For this review, take the finished solid that the model builds, in its own axes (mm). A direction names the side the tool comes from. Round coordinates to 2 decimals unless told otherwise and drop trailing zeros. Loops run counter-clockwise (first coordinate to the right, second up) from the corner with the lowest first, then second, coordinate; pieces in that order, holes last. Notation, with made-up numbers: M 19.5,-21.5 L 62.5,-21.5 A28 cw 62.5,10.5 Z; hole C 23.25,68 d10. An arc over 180 degrees is marked long. Write item = value, one per line. Start each with the question number.
```python
from build123d import *

# Parameters (mm, degrees)
SKETCH1_W               = 119
SKETCH1_H               = 50
BOSS_EXTRUDE1_DEPTH     = 95
SKETCH2_W               = 115
SKETCH2_H               = 46
CUT_EXTRUDE1_DEPTH      = 92
SKETCH3_W               = 50
SKETCH3_H               = 29
CUT_EXTRUDE2_DEPTH      = 10
SKETCH4_R               = 1.95
CUT_EXTRUDE3_DEPTH      = 10
SKETCH5_R               = 3.25
SKETCH5_R_2             = 1.95
BOSS_EXTRUDE3_DEPTH     = 10
FILLET1_R               = 2
SKETCH6_R               = 2
CUT_EXTRUDE4_DEPTH      = 10
CUT_EXTRUDE5_DEPTH      = 159.789168456
CUT_EXTRUDE5_DEPTH_BACK = 159.789168456
SKETCH8_R               = 2
BOSS_EXTRUDE4_DEPTH     = 115
CUT_EXTRUDE6_DEPTH      = 159.789168456
CUT_EXTRUDE6_DEPTH_BACK = 159.789168456
CUT_EXTRUDE8_DEPTH      = 10
CUT_EXTRUDE9_DEPTH      = 155.550962524


with BuildPart() as part:
    # Sketch1 → Boss-Extrude1 (new body)
    with BuildSketch(Plane.XY):
        with Locations((59.5, 25)):
            Rectangle(SKETCH1_W, SKETCH1_H)
    extrude(amount=BOSS_EXTRUDE1_DEPTH)

    # Sketch2 → Cut-Extrude1 (cut)
    with BuildSketch(Plane.XY.offset(95)):
        with Locations((59.5, 25)):
            Rectangle(SKETCH2_W, SKETCH2_H)
    extrude(amount=-CUT_EXTRUDE1_DEPTH, mode=Mode.SUBTRACT)

    # Sketch3 → Cut-Extrude2 (cut)
    with BuildSketch(Plane.XY.offset(3)):
        with Locations((33, 25)):
            Rectangle(SKETCH3_W, SKETCH3_H)
    extrude(amount=-CUT_EXTRUDE2_DEPTH, mode=Mode.SUBTRACT)

    # Sketch4 → Cut-Extrude3 (cut)
    with BuildSketch(Plane(origin=(0, 0, 0), x_dir=(-1, 0, 0), z_dir=(0, 0, -1))):
        with Locations((-32.95, 45)):
            Circle(SKETCH4_R)
        with Locations((-32.95, 5)):
            Circle(SKETCH4_R)
    extrude(amount=-CUT_EXTRUDE3_DEPTH, mode=Mode.SUBTRACT)

    # Sketch5 → Boss-Extrude3 (add)
    # profile 1 of 2: a face of its own
    with BuildSketch(Plane.XY.offset(3)):
        with Locations((32.95, 45)):
            Circle(SKETCH5_R)
        with Locations(Location((32.95, 45, 0), (0, 0, 180))):
            Circle(SKETCH5_R_2, mode=Mode.SUBTRACT)
    # profile 2 of 2: a face of its own
    with BuildSketch(Plane.XY.offset(3)):
        with Locations((32.95, 5)):
            Circle(SKETCH5_R)
        with Locations(Location((32.95, 5, 0), (0, 0, 180))):
            Circle(SKETCH5_R_2, mode=Mode.SUBTRACT)
    extrude(amount=BOSS_EXTRUDE3_DEPTH)

    # Fillet1
    fillet1_edges = [part.edges().sort_by_distance(p)[0] for p in [
        (31.147224362, 42.295836543, 3),
        (31.147224362, 7.704163457, 3),
    ]]
    fillet(fillet1_edges, radius=FILLET1_R)

    # Sketch6 → Cut-Extrude4 (cut)
    with BuildSketch(Plane(origin=(0, 2, 0), x_dir=(1, 0, 0), z_dir=(0, 1, 0))):
        with Locations(Location((85, -90, 0), (0, 0, 180))):
            Circle(SKETCH6_R)
        with Locations(Location((35, -90, 0), (0, 0, 180))):
            Circle(SKETCH6_R)
    extrude(amount=-CUT_EXTRUDE4_DEPTH, mode=Mode.SUBTRACT)

    # Sketch8 → Cut-Extrude5 (cut, two sides: drawn at the far end of the back side and taken through both)
    with BuildSketch(Plane(origin=(2, 0, 0), x_dir=(0, 0, -1), z_dir=(1, 0, 0)).offset(-CUT_EXTRUDE5_DEPTH_BACK)):
        with Locations(Location((-90, 14.5, 0), (0, 0, 90))):
            Circle(SKETCH8_R)
    extrude(amount=CUT_EXTRUDE5_DEPTH + CUT_EXTRUDE5_DEPTH_BACK, mode=Mode.SUBTRACT)

    # Sketch9 → Boss-Extrude4 (add)
    with BuildSketch(Plane(origin=(2, 0, 0), x_dir=(0, 0, -1), z_dir=(1, 0, 0))):
        Polygon((-95, 33), (-73.577779899, 48), (-71.577779899, 48), (-93, 33), align=None)
    extrude(amount=BOSS_EXTRUDE4_DEPTH)

    # Sketch10 → Cut-Extrude6 (cut, two sides: drawn at the far end of the back side and taken through both)
    with BuildSketch(Plane(origin=(2, 0, 0), x_dir=(0, 0, -1), z_dir=(1, 0, 0)).offset(-CUT_EXTRUDE6_DEPTH_BACK)):
        Polygon((-95, 33), (-95, 50), (-70.721483885, 50), align=None)
    extrude(amount=CUT_EXTRUDE6_DEPTH + CUT_EXTRUDE6_DEPTH_BACK, mode=Mode.SUBTRACT)

    # Sketch11 → Cut-Extrude8 (cut)
    with BuildSketch(Plane(origin=(0, 0, 0), x_dir=(-1, 0, 0), z_dir=(0, 0, -1))):
        with BuildLine():
            Line((-109.202811856, 45), (-109.202811856, 5))
            ThreePointArc((-109.202811856, 5), (-111, 3.202811856), (-112.797188144, 5))
            Line((-112.797188144, 5), (-112.797188144, 45))
            ThreePointArc((-112.797188144, 45), (-111, 46.797188144), (-109.202811856, 45))
        make_face()
        with BuildLine():
            Line((-102.202811856, 45), (-102.202811856, 5))
            ThreePointArc((-102.202811856, 5), (-104, 3.202811856), (-105.797188144, 5))
            Line((-105.797188144, 5), (-105.797188144, 45))
            ThreePointArc((-105.797188144, 45), (-104, 46.797188144), (-102.202811856, 45))
        make_face()
        with BuildLine():
            Line((-95.202811856, 45), (-95.202811856, 5))
            ThreePointArc((-95.202811856, 5), (-97, 3.202811856), (-98.797188144, 5))
            Line((-98.797188144, 5), (-98.797188144, 45))
            ThreePointArc((-98.797188144, 45), (-97, 46.797188144), (-95.202811856, 45))
        make_face()
        with BuildLine():
            Line((-88.202811856, 45), (-88.202811856, 5))
            ThreePointArc((-88.202811856, 5), (-90, 3.202811856), (-91.797188144, 5))
            Line((-91.797188144, 5), (-91.797188144, 45))
            ThreePointArc((-91.797188144, 45), (-90, 46.797188144), (-88.202811856, 45))
        make_face()
        with BuildLine():
            Line((-81.202811856, 45), (-81.202811856, 5))
            ThreePointArc((-81.202811856, 5), (-83, 3.202811856), (-84.797188144, 5))
            Line((-84.797188144, 5), (-84.797188144, 45))
            ThreePointArc((-84.797188144, 45), (-83, 46.797188144), (-81.202811856, 45))
        make_face()
        with BuildLine():
            Line((-74.202811856, 45), (-74.202811856, 5))
            ThreePointArc((-74.202811856, 5), (-76, 3.202811856), (-77.797188144, 5))
            Line((-77.797188144, 5), (-77.797188144, 45))
            ThreePointArc((-77.797188144, 45), (-76, 46.797188144), (-74.202811856, 45))
        make_face()
        with BuildLine():
            Line((-67.202811856, 45), (-67.202811856, 5))
            ThreePointArc((-67.202811856, 5), (-69, 3.202811856), (-70.797188144, 5))
            Line((-70.797188144, 5), (-70.797188144, 45))
            ThreePointArc((-70.797188144, 45), (-69, 46.797188144), (-67.202811856, 45))
        make_face()
    extrude(amount=-CUT_EXTRUDE8_DEPTH, mode=Mode.SUBTRACT)

    # Sketch12 → Cut-Extrude9 (cut, through all)
    with BuildSketch(Plane.XY.offset(10)):
        with BuildLine():
            Line((108.667383108, 29), (91.910743178, 29))
            ThreePointArc((91.910743178, 29), (87.910743178, 33), (91.910743178, 37))
            Line((91.910743178, 37), (108.667383108, 37))
            ThreePointArc((108.667383108, 37), (112.667383108, 33), (108.667383108, 29))
        make_face()
    extrude(amount=CUT_EXTRUDE9_DEPTH, mode=Mode.SUBTRACT)


solid = part.part
```
(1) Draft analysis for pull direction Y (two halves, no side actions). For faces 5 (the flat face through (59, 2, 50)), 6 (the flat face through (0, 25, 47)), 7 (the flat face through (59, 50, 35)), state which applies: +Y half, -Y half, draft (parallel to the pull), parting line (faces both ways), or undercut.
(2) Tool access review of faces 1 (the flat face through (8, 25, 2)), 2 (the flat face through (46, 41, 3)), 3 (the flat face through (34, 7, 13)), 4 (the cylindrical face through (96.96, 3.203, 1.479)): name each direction out of +Z, -Z, +X, -X, +Y, -Y from which nothing blocks a thin tool from reaching the whole face with its end or side.
(3) Add section B-B on z = 10. Write out the cut boundary in (x, y), and give its area (3 significant figures).
(4) Add section D-D on y = 20. Count the separate pieces of the cut face and the enclosed holes in it, and give its area (3 significant figures).
(5) Wall thickness on L1, parallel to X at y = 20, z = 58; L2, parallel to Y at x = 104, z = 31; L3, parallel to X at y = 45, z = 4.75: over which ranges is each line inside the solid? List them lowest first.
(6) Add section A-A on x = 69. Write out the cut boundary in (y, z).
(7) Add section C-C on z = 40. Write out the cut boundary in (x, y).
Answer sheet:
q1.face_5 = undercut
q1.face_6 = draft
q1.face_7 = +Y half
q2.face_1 = -Z
q2.face_2 = none
q2.face_3 = +Z
q2.face_4 = +Z, -Z
q3.outline = M 0,0 L 119,0 L 119,50 L 0,50 Z; hole M 2,2 L 31.7,2 A3.25 cw long 34.2,2 L 117,2 L 117,48 L 34.2,48 A3.25 cw long 31.7,48 L 2,48 Z; hole C 32.95,5 d3.9; hole C 32.95,45 d3.9
q3.area = 702 mm²
q4.separate_pieces = 9
q4.enclosed_holes = 0
q4.area = 500 mm²
q5.L1 = 0 to 2, 117 to 119
q5.L2 = 0 to 2, 48 to 50
q5.L3 = 0 to 2, 29.68 to 31, 34.9 to 36.22, 117 to 119
q6.outline = M 0,0 L 3.2,0 L 3.2,3 L 2,3 L 2,95 L 0,95 Z; M 33,93 L 48,71.58 L 48,3 L 46.8,3 L 46.8,0 L 50,0 L 50,70.72 L 33,95 Z
q7.outline = M 0,0 L 119,0 L 119,50 L 0,50 Z; hole M 2,2 L 117,2 L 117,48 L 2,48 Z
